Check sheet for the modelled part. Datum: model origin and axes. Units: mm. A direction names the side the tool comes from. Round coordinates to 2 decimals unless told otherwise and drop trailing zeros. Write each loop counter-clockwise with the first axis right and the second up, starting at its lowest first coordinate (ties: lowest second). Pieces come first, ordered by that corner, then holes. Notation, with made-up numbers: M 1.25,-11.75 L 11.25,-11.75 A21 ccw 11.25,26.25 Z; hole C -40,-26 d1. An arc over 180 degrees is marked long. Answer in a Markdown table with one row per item.
Autodesk Inventor part; units mm, degrees
ref_plane "YZ Plane" through (0, 0, 0) normal (1, 0, 0) x (0, 1, 0)
ref_plane "XZ Plane" through (0, 0, 0) normal (0, 1, 0) x (-1, 0, 0)
ref_plane "XY Plane" through (0, 0, 0) normal (0, 0, 1) x (1, 0, 0)
sketch "Sketch1" plane through (0, 0, 0) normal (0, 1, 0) x (-1, 0, 0)
  line L0 (75.0098, 31.2127) -> (69.5098, 31.2127)
  line L1 (75.0098, 31.2127) -> (80.5098, 31.2127) construction
  line L2 (69.5098, 31.2127) -> (69.5098, 11.2127)
  line L3 (69.5098, 11.2127) -> (75.0098, 11.2127)
  line L4 (75.0098, -11.213) -> (69.5098, -11.213)
  line L5 (69.5098, -11.213) -> (69.5098, -31.213)
  line L6 (69.5098, -31.213) -> (75.0098, -31.213)
  line L7 (75.0098, -31.213) -> (75.0098, -43.3013)
  line L8 (75.0098, 43.3013) -> (75.0098, 31.2127)
  line L9 (75.0098, 11.2127) -> (75.0098, -11.213)
  line L10 (64.5408, -49.3456) -> (61.7908, -44.5824)
  line L11 (64.5408, -49.3456) -> (67.2908, -54.1087) construction
  line L12 (61.7908, -44.5824) -> (44.4702, -54.5824)
  line L13 (44.4702, -54.5824) -> (47.2202, -59.3456)
  line L14 (27.799, -70.5584) -> (25.049, -65.7953)
  line L15 (25.049, -65.7953) -> (7.7285, -75.7953)
  line L16 (7.7285, -75.7953) -> (10.4785, -80.5584)
  line L17 (10.4785, -80.5584) -> (0.0098, -86.6025)
  line L18 (75.0098, -43.3013) -> (64.5408, -49.3456)
  line L19 (47.2202, -59.3456) -> (27.799, -70.5584)
  line L20 (-10.4592, -80.5582) -> (-7.7092, -75.7951)
  line L21 (-10.4592, -80.5582) -> (-13.2092, -85.3214) construction
  line L22 (-7.7092, -75.7951) -> (-25.0298, -65.7951)
  line L23 (-25.0298, -65.7951) -> (-27.7798, -70.5582)
  line L24 (-47.201, -59.3454) -> (-44.451, -54.5823)
  line L25 (-44.451, -54.5823) -> (-61.7715, -44.5823)
  line L26 (-61.7715, -44.5823) -> (-64.5215, -49.3454)
  line L27 (-64.5215, -49.3454) -> (-74.9902, -43.3013)
  line L28 (0.0098, -86.6025) -> (-10.4592, -80.5582)
  line L29 (-27.7798, -70.5582) -> (-47.201, -59.3454)
  line L30 (-74.9902, -31.2127) -> (-69.4902, -31.2127)
  line L31 (-74.9902, -31.2127) -> (-80.4902, -31.2127) construction
  line L32 (-69.4902, -31.2127) -> (-69.4902, -11.2127)
  line L33 (-69.4902, -11.2127) -> (-74.9902, -11.2127)
  line L34 (-74.9902, 11.213) -> (-69.4902, 11.213)
  line L35 (-69.4902, 11.213) -> (-69.4902, 31.213)
  line L36 (-69.4902, 31.213) -> (-74.9902, 31.213)
  line L37 (-74.9902, 31.213) -> (-74.9902, 43.3013)
  line L38 (-74.9902, -43.3013) -> (-74.9902, -31.2127)
  line L39 (-74.9902, -11.2127) -> (-74.9902, 11.213)
  line L40 (-64.5212, 49.3456) -> (-61.7712, 44.5824)
  line L41 (-64.5212, 49.3456) -> (-67.2712, 54.1087) construction
  line L42 (-61.7712, 44.5824) -> (-44.4507, 54.5824)
  line L43 (-44.4507, 54.5824) -> (-47.2007, 59.3456)
  line L44 (-27.7795, 70.5584) -> (-25.0295, 65.7953)
  line L45 (-25.0295, 65.7953) -> (-7.709, 75.7953)
  line L46 (-7.709, 75.7953) -> (-10.459, 80.5584)
  line L47 (-10.459, 80.5584) -> (0.0098, 86.6025)
  line L48 (-74.9902, 43.3013) -> (-64.5212, 49.3456)
  line L49 (-47.2007, 59.3456) -> (-27.7795, 70.5584)
  line L50 (10.4788, 80.5582) -> (7.7288, 75.7951)
  line L51 (10.4788, 80.5582) -> (13.2288, 85.3214) construction
  line L52 (7.7288, 75.7951) -> (25.0493, 65.7951)
  line L53 (25.0493, 65.7951) -> (27.7993, 70.5582)
  line L54 (47.2205, 59.3454) -> (44.4705, 54.5823)
  line L55 (44.4705, 54.5823) -> (61.791, 44.5823)
  line L56 (61.791, 44.5823) -> (64.541, 49.3454)
  line L57 (64.541, 49.3454) -> (75.0098, 43.3013)
  line L58 (0.0098, 86.6025) -> (10.4788, 80.5582)
  line L59 (27.7993, 70.5582) -> (47.2205, 59.3454)
  line L60 (64.541, 49.3454) -> (75.0098, 43.3013)
  line L61 (0.0098, 86.6025) -> (10.4788, 80.5582)
  line L62 (27.7993, 70.5582) -> (47.2205, 59.3454)
  line L63 (-10.459, 80.5584) -> (0.0098, 86.6025)
  line L64 (-74.9902, 43.3013) -> (-64.5212, 49.3456)
  line L65 (-47.2007, 59.3456) -> (-27.7795, 70.5584)
  line L66 (-74.9902, 31.213) -> (-74.9902, 43.3013)
  line L67 (-74.9902, -43.3013) -> (-74.9902, -31.2127)
  line L68 (-74.9902, -11.2127) -> (-74.9902, 11.213)
  line L69 (-64.5215, -49.3454) -> (-74.9902, -43.3013)
  line L70 (0.0098, -86.6025) -> (-10.4592, -80.5582)
  line L71 (-27.7798, -70.5582) -> (-47.201, -59.3454)
  line L72 (10.4785, -80.5584) -> (0.0098, -86.6025)
  line L73 (75.0098, -43.3013) -> (64.5408, -49.3456)
  line L74 (47.2202, -59.3456) -> (27.799, -70.5584)
  point P0 (0.0098, 0)
  point P1 (0.0098, 0)
  point P2 (0.0098, 0)
  point P3 (0.0098, 0)
  point P4 (0.0098, 0)
  point P5 (0.0098, 0)
  dimension "d6" = 86.6025
  dimension "d7" = 5.5
  dimension "d8" = 180
  dimension "d9" = 20
  dimension "d10" = 20
  dimension "d13" = 360
extrude "Extrusion1" add sketch "Sketch1" along normal blind 5.5
sketch "Sketch2" plane through (0, 0, 0) normal (0, -1, 0) x (1, 0, 0)
  line L0 (-17.3205, -10) -> (-25.9808, -15)
  line L1 (-25.9808, -15) -> (-24.9808, -16.7321)
  line L2 (-24.9808, -16.7321) -> (-16.3205, -11.7321)
  line L3 (-16.3205, -11.7321) -> (-17.3205, -10)
  line L4 (17.3205, 10) -> (25.9808, 15)
  line L5 (25.9808, 15) -> (26.9808, 13.2679)
  line L6 (26.9808, 13.2679) -> (18.3205, 8.2679)
  line L7 (18.3205, 8.2679) -> (17.3205, 10)
  point P0 (0, 0)
  dimension "d17" = 10
  dimension "d18" = 2
  dimension "d19" = 10
  dimension "d22" = 20
  dimension "d23" = 20
extrude "Extrusion2" cut sketch "Sketch2" against normal blind 10
sketch "Sketch4" plane through (0, 0, 0) normal (0, -1, 0) x (1, 0, 0)
  line L0 (13.9904, 5.7679) -> (9.6603, 3.2679)
  line L1 (9.6603, 3.2679) -> (12.4103, -1.4952)
  line L2 (12.4103, -1.4952) -> (16.7404, 1.0048)
  line L3 (16.7404, 1.0048) -> (13.9904, 5.7679)
  line L4 (31.3109, 15.7679) -> (35.641, 18.2679)
  line L5 (35.641, 18.2679) -> (38.391, 13.5048)
  line L6 (38.391, 13.5048) -> (34.0609, 11.0048)
  line L7 (34.0609, 11.0048) -> (31.3109, 15.7679)
  line L8 (-11.9904, -9.2321) -> (-7.6603, -6.7321)
  line L9 (-7.6603, -6.7321) -> (-4.9103, -11.4952)
  line L10 (-4.9103, -11.4952) -> (-9.2404, -13.9952)
  line L11 (-9.2404, -13.9952) -> (-11.9904, -9.2321)
  line L12 (-29.3109, -19.2321) -> (-33.641, -21.7321)
  line L13 (-33.641, -21.7321) -> (-30.891, -26.4952)
  line L14 (-30.891, -26.4952) -> (-26.5609, -23.9952)
  line L15 (-26.5609, -23.9952) -> (-29.3109, -19.2321)
  point P0 (0, 0)
  dimension "d24" = 5
  dimension "d25" = 5.5
  dimension "d26" = 5
  dimension "d27" = 5.5
extrude "Extrusion3" cut sketch "Sketch4" against normal blind 10
properties part number "base"
1. Scan lines: L1, parallel to X at y = 1.95, z = 70; L2, parallel to X at y = 3.25, z = 68; L3, parallel to X at y = 3.4, z = -27.5. Record each from-to range of solid material in increasing order.
Found:
| item | result |
|---|---|
| L1 | x = -28.77 to -27.48, -17.77 to 17.75, 27.46 to 28.75 |
| L2 | x = -32.23 to -26.32, -21.23 to 21.21, 26.3 to 32.21 |
| L3 | x = -69.51 to 69.49 |
2. Draft check along X on faces 1 (the face through (-72, 3, -31.213)), 2 (the face through (16.248, 2.712, -70.865)), 3 (the face through (-5.317, 2.712, -83.538)). Enter one of: +X half, -X half, draft (parallel to the pull), parting line (faces both ways), or undercut.
Found:
| item | result |
|---|---|
| face 1 | draft |
| face 2 | undercut |
| face 3 | -X half |
3. Section check D-D, the plane x = 3.5. Record the cut outline in (y, z).
Found:
| item | result |
|---|---|
| outline | M 0,-84.58 L 5.5,-84.58 L 5.5,84.58 L 0,84.58 Z |
4. Go/stop test with flat-tipped pins: pin 1 (1.6 mm diameter, centred on x = 73, y = 1.5, fed in from -Z); pin 2 (2 mm diameter, centred on x = -17.5, y = 1.5, fed in from -Z); pin 3 (1.6 mm diameter, centred on x = 72.5, y = 2, fed in from +Z); pin 4 (4 mm diameter, centred on x = 17, z = 10, fed in from -Y). Record where each tip stops, or that it passes through.
Found:
| item | result |
|---|---|
| pin 1 | stops at z = -44.91 |
| pin 2 | stops at z = -70.73 |
| pin 3 | stops at z = 45.2 |
| pin 4 | stops at y = 0 |
5. Access from +Z, -Z, +X, -X, +Y, -Y to the whole of each face (thin tool, end or side, straight path). Record for faces 4 (the face through (-63.185, 2.712, -46.997)), 5 (the face through (9.065, 2.712, 78.144)), 6 (the face through (-72, 3, 11.213)), 7 (the face through (-10.596, 2.712, -11.647)).
Found:
| item | result |
|---|---|
| face 4 | -Z, +Y, -Y |
| face 5 | +X, +Y, -Y |
| face 6 | -X, +Y, -Y |
| face 7 | +Y, -Y |
6. Section check B-B, the plane y = 3.35. Count the separate pieces of the cut face and the enclosed holes in it, and give its area (3 significant figures).
Found:
| item | result |
|---|---|
| separate pieces | 1 |
| enclosed holes | 6 |
| area | 18,000 mm2 |
7. Section check C-C, the plane z = -56.5. Record the cut outline in (x, y).
Found:
| item | result |
|---|---|
| outline | M -45.58,0 L 45.56,0 L 45.56,5.5 L -45.58,5.5 Z |
8. Section check A-A, the plane x = -22. Record the cut outline in (y, z).
Found:
| item | result |
|---|---|
| outline | M 0,-67.56 L 5.5,-67.56 L 5.5,-15.01 L 0,-15.01 Z; M 0,-12.7 L 5.5,-12.7 L 5.5,67.56 L 0,67.56 Z |
